The figure shows three views and two pictorial views of one solid part (mm, origin at its lowest corner). Answer the questions. Coordinates: 2 decimals unless noted, no trailing zeros. Loops run counter-clockwise (first coordinate to the right, second up) from the corner with the lowest first, then second, coordinate; pieces in that order, holes last. Notation, with made-up numbers: (-21.75, 19.25) -> (-16.75, 19.25) arc R33 ccw to (-16.75, 55.25) -> close; hole circle Ø10 at (4, 49.5). An arc over 180 degrees is marked (long way). Answer as a JSON object with one key per item and string values. Group by question number.
1) Section B-B, the plane x = 10 is taken. Give the vertices of the cut face in (y, z), plus the area to 3 significant figures.
2) Section C-C, the plane z = 0.45 is taken. Give the vertices of the cut face in (x, y), plus the area to 3 significant figures.
3) Flat-ended cylindrical pins translate along their axes: P1, Ø1.3, axis at x = 1.5, y = 11, coming from the +Z side; P2, Ø1, axis at y = 17, z = 0.5, coming from the +X side; P3, Ø1.5, axis at x = 17, z = 2.5, coming from the +Y side; P4, Ø5, axis at x = 11, y = 7, coming from the +Z side. Find the tip coordinate at first contact, or state that the pin passes through.
4) Consider probe 1 along X at (y, z) = (10, 1.8); probe 2 along X at (y, z) = (10, 2.2). Determine where each line is inside the solid, lowest interval first. Write a range as [from, to].
5) Section A-A, the plane y = 10 is taken. Give the vertices of the cut face in (x, z), plus the area to 3 significant figures.
6) Section D-D, the plane x = 3.75 is taken. Give the vertices of the cut face in (y, z), plus the area to 3 significant figures.
7) Determine the mould class of the marked faces 1, 2, 3 and 4 for opening direction Y: released by +Y, released by -Y, zero draft, split by the parting line, or undercut.
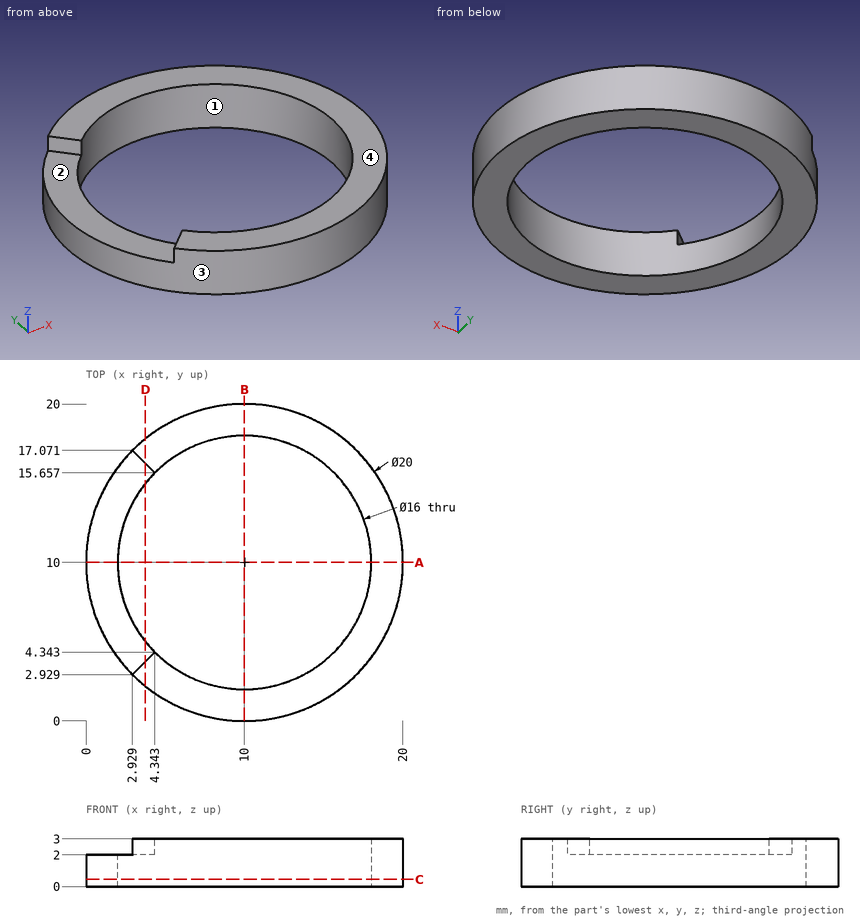
Determined:
{
 "1": {"outline": "(0, 0) -> (2, 0) -> (2, 3) -> (0, 3) -> close; (18, 0) -> (20, 0) -> (20, 3) -> (18, 3) -> close", "area": "12.0 mm²"},
 "2": {"outline": "circle Ø20 at (10, 10); hole circle Ø16 at (10, 10)", "area": "113 mm²"},
 "3": {"P1": "z = 2", "P2": "x = 17.6", "P3": "y = 17.81", "P4": "through"},
 "4": {"probe 1": "[0, 2], [18, 20]", "probe 2": "[18, 20]"},
 "5": {"outline": "(0, 0) -> (2, 0) -> (2, 2) -> (0, 2) -> close; (18, 0) -> (20, 0) -> (20, 3) -> (18, 3) -> close", "area": "10.0 mm²"},
 "6": {"outline": "(2.19, 0) -> (5.01, 0) -> (5.01, 2) -> (3.75, 2) -> (3.75, 3) -> (2.19, 3) -> close; (14.99, 0) -> (17.81, 0) -> (17.81, 3) -> (16.25, 3) -> (16.25, 2) -> (14.99, 2) -> close", "area": "14.4 mm²"},
 "7": {"face 1": "undercut", "face 2": "undercut", "face 3": "split by the parting line", "face 4": "zero draft"}
}
